from build123d import *

# Parameters (mm, degrees)
ESTRUSIONE_ESTRUSIONE1_DEPTH = 5
SCHIZZO2_R                   = 2
TAGLIO_ESTRUSIONE1_DEPTH     = 6


with BuildPart() as part:
    # Schizzo1 → Estrusione-Estrusione1 (new body)
    with BuildSketch(Plane(origin=(0, 0, 0), x_dir=(0, 0, -1), z_dir=(1, 0, 0))):
        with BuildLine():
            Line((-50, 15), (50, 15))
            ThreePointArc((50, 15), (65, 0), (50, -15))
            Line((50, -15), (-50, -15))
            ThreePointArc((-50, -15), (-65, 0), (-50, 15))
        make_face()
    extrude(amount=ESTRUSIONE_ESTRUSIONE1_DEPTH)

    # Schizzo2 → Taglio-Estrusione1 (cut, through all)
    with BuildSketch(Plane(origin=(5, 0, 0), x_dir=(0, 0, -1), z_dir=(1, 0, 0))):
        with Locations((-50, 0)):
            Circle(SCHIZZO2_R)
        Circle(SCHIZZO2_R)
        with Locations((50, 0)):
            Circle(SCHIZZO2_R)
    extrude(amount=-TAGLIO_ESTRUSIONE1_DEPTH, mode=Mode.SUBTRACT)


solid = part.part
Build history of the part. All positions in model axes, mm. Coordinates: 2 decimals unless noted, no trailing zeros. Write each loop counter-clockwise with the first axis right and the second up, starting at its lowest first coordinate (ties: lowest second). Pieces come first, ordered by that corner, then holes.
(1) Cut at D-D on y = 11.5. List the corners of the cut face in (x, z), and give its area (3 significant figures).
(2) Cut at A-A on y = 0. List the corners of the cut face in (x, z).
(3) Mould opens along Z. For faces 1 (the cylindrical face through (2, 0, -65)), 2 (the cylindrical face through (2, 0, 65)), 3 (the cylindrical face through (3, -2, 0)) say: pulls with the +Z half, pulls with the -Z half, needs draft (parallel to the pull), parting line crosses it, or undercut.
(4) Drill centre lines: line 1 (Y direction, x = 4.05, z = 50); line 2 (Z direction, x = 3.9, y = -5); line 3 (Z direction, x = 2.6, y = 5.5). Where is each one in solid material? Low to high.
(5) Cut at C-C on x = 4.1. List the corners of the cut face in (y, z).
(6) Cut at B-B on z = 0. List the corners of the cut face in (x, y).
Working result:
1. outline: (0, -59.63) - (5, -59.63) - (5, 59.63) - (0, 59.63) - close
1. area: 596 mm2
2. outline: (0, -65) - (5, -65) - (5, -52) - (0, -52) - close; (0, -48) - (5, -48) - (5, -2) - (0, -2) - close; (0, 2) - (5, 2) - (5, 48) - (0, 48) - close; (0, 52) - (5, 52) - (5, 65) - (0, 65) - close
3. face 1: pulls with the -Z half
3. face 2: pulls with the +Z half
3. face 3: undercut
4. line 1: y = -15 to -2, 2 to 15
4. line 2: z = -64.14 to 64.14
4. line 3: z = -63.96 to 63.96
5. outline: (-15, -50) arc R15 ccw to (15, -50) - (15, 50) arc R15 ccw to (-15, 50) - close; hole circle Ø4 at (0, -50); hole circle Ø4 at (0, 0); hole circle Ø4 at (0, 50)
6. outline: (0, -15) - (5, -15) - (5, -2) - (0, -2) - close; (0, 2) - (5, 2) - (5, 15) - (0, 15) - close
